The listing builds one solid part. Answer for the finished solid, in the listing's coordinates (mm). Give positions to 0.01 mm unless a question says otherwise; leave off trailing zeros. Loops run counter-clockwise (first coordinate to the right, second up) from the corner with the lowest first, then second, coordinate; pieces in that order, holes last.
Item 1: Consider line 1 along Z through (x, y) = (3.3, 61); line 2 along Y through (x, z) = (1.8, 212.5). Determine where each line is inside the solid, lowest interval first.
Item 2: Each of these flat-tipped pins is pushed along its axis until it touches: pin 1 Ø2 at (x, z) = (3, 263.5) entering from -Y; pin 2 Ø1.2 at (x, y) = (1, 348) entering from +Z; pin 3 Ø1.2 at (x, z) = (1.5, 23) entering from +Y. Where does it stop, or does it pass through?
Item 3: Section A-A, the plane z = 74 is taken. Give the vertices of the cut face in (x, y), and give its area (3 significant figures).
Autodesk Fusion 360 part; units mm, degrees
sketch "Sketch1" plane through (0, 0, 0) normal (1, 0, 0) x (0, 1, 0)
  line L0 (0, 0) -> (350, 0)
  line L1 (350, 0) -> (350, 280)
  line L2 (350, 280) -> (0, 280)
  line L3 (0, 280) -> (0, 0)
  line L4 (0, 276) -> (4, 276)
  line L5 (4, 276) -> (4, 246)
  line L6 (4, 246) -> (0, 246)
  line L7 (0, 246) -> (0, 276)
  line L8 (40, 280) -> (70, 280)
  line L9 (70, 280) -> (70, 276)
  line L10 (70, 276) -> (40, 276)
  line L11 (40, 276) -> (40, 280)
  line L12 (0, 280) -> (10, 280)
  line L13 (10, 280) -> (10, 276)
  line L14 (10, 276) -> (0, 276)
  line L15 (0, 276) -> (0, 280)
  dimension "d5" = 350
  dimension "d6" = 280
  dimension "d7" = 30
  dimension "d8" = 30
  dimension "d9" = 4
  dimension "d10" = 4
  dimension "d14" = 10
  dimension "d15" = 4
  dimension "d16" = 30
extrude "Extrude1" add sketch "Sketch1" along normal blind 4 makes body 1
extrude "Extrude2" cut sketch "Sketch1" along normal through all contours L3 L4 L5 L6 L7 L14 bodies 1
extrude "Extrude3" cut sketch "Sketch1" along normal through all contours L2 L3 L4 L12 L13 L14 L15 bodies 1
extrude "Extrude4" cut sketch "Sketch1" along normal through all contours L2 L8 L9 L10 L11 bodies 1
pattern_linear "R-Pattern1" count 5 spacing 60 along (0, 0, -1) count 2 spacing 346 along (0, 1, 0) of "Extrude2"
pattern_linear "R-Pattern2" count 2 spacing 340 along (0, 1, 0) of "Extrude3"
pattern_linear "R-Pattern3" count 5 spacing 60 along (0, 1, 0) of "Extrude4"
copy_body "Body->Comp1" bodies 1 removing the originals makes body 2 in component "Component"
component "Component" placed x (1, 0, 0) y (0, 1, 0) z (0, 0, 1) at (0, 0, 0)
equation "d5 = Linear Dimension-2"
equation "d6 = Linear Dimension-3"
equation "d9 = Linear Dimension-6"
equation "d10 = Linear Dimension-7"
equation "a_d = ( d - floor(d / a) * a ) / 2"
equation "d14 = a_d"
equation "d15 = Linear Dimension-11"
equation "d16 = Linear Dimension-11"
equation "d27 = a * 2"
equation "d28 = d - t"
equation "d31 = d - a_d"
equation "d35 = 2 * a"
Worked answers:
1. line 1: z = 0 to 276
1. line 2: y = 4 to 346
2. pin 1: stops at y = 4
2. pin 2: stops at z = 246
2. pin 3: stops at y = 346
3. outline: (0, 4) - (4, 4) - (4, 346) - (0, 346) - close
3. area: 1,370 mm2
